The listing builds one solid part. Answer for the finished solid, in the listing's coordinates (mm). A direction names the side the tool comes from. Coordinates: 2 decimals unless noted, no trailing zeros. Loops run counter-clockwise (first coordinate to the right, second up) from the corner with the lowest first, then second, coordinate; pieces in that order, holes last. Notation, with made-up numbers: (85.5, 42.25) -> (137.5, 42.25) arc R15 cw to (137.5, 56.25) -> close; hole circle Ø1 at (48, 68.5). An arc over 180 degrees is marked (long way). Answer in a Markdown table with one row per item.
```python
from build123d import *

# Parameters (mm, degrees)
F0_W     = 38.1
F0_H     = 605.4239357613
F0_H_2   = 901.7
F0_W_2   = 121.1758604333
F0_H_3   = 38.1
F1_DEPTH = 88.9


# Not quite as in the source:
# - a feature names something its author has since deleted; it is built from what else it names


with BuildPart() as f1:
    # F0 (on Front) → F1 (new body)
    with BuildSketch(Plane.XZ):
        Polygon((0, 38.1), (0, 0), (558.8, 0), (558.8, 38.1), (520.7027813, 38.1), (399.5269208667, 38.1), (361.4269208667, 38.1), (218.8134604333, 38.1), (180.7134604333, 38.1), (38.1, 38.1), align=None)
        with Locations((19.05, 340.8119678807)):
            Rectangle(F0_W, F0_H)
        Polygon((520.7027813, 38.1), (558.8, 38.1), (558.8027813, 38.1), (558.8027813, 939.8), (558.8027813, 1181.4738530943), (558.8027813, 1235.3553898208), (558.8027813, 1270), (520.7027813, 1270), (520.7027813, 977.9), (520.7027813, 939.8), align=None)
        Polygon((69.5237996219, 939.8), (0, 643.5239357613), (38.1, 643.5239357613), (39.1349278428, 643.5239357613), (108.6587274647, 939.8), align=None)
        with Locations((199.7634604333, 488.95)):
            Rectangle(F0_W, F0_H_2)
        Polygon((96.2017068277, 977.9), (69.5237996219, 939.8), (108.6587274647, 939.8), (180.7134604333, 939.8), (218.8134604333, 939.8), (361.4269208667, 939.8), (361.4269208667, 977.9), (142.7132186595, 977.9), align=None)
        Polygon((361.4269208667, 38.1), (399.5269208667, 38.1), (399.5269208667, 939.8), (399.5269208667, 977.9), (399.5269208667, 1270), (361.4269208667, 1270), (361.4269208667, 977.9), (361.4269208667, 939.8), align=None)
        with Locations((460.1148510833, 958.85)):
            Rectangle(F0_W_2, F0_H_3)
        Polygon((300.7323287388, 1270), (96.2017068277, 977.9), (142.7132186595, 977.9), (347.2438405706, 1270), align=None)
        Polygon((558.8027813, 1235.3553898208), (558.8027813, 1181.4738530943), (774.3289282057, 1397), (720.4473914792, 1397), align=None)
        Polygon((338.8323287388, 1308.1), (300.7323287388, 1270), (347.2438405706, 1270), (361.4269208667, 1270), (399.5269208667, 1270), (520.7027813, 1270), (558.8027813, 1270), (558.8027813, 1308.1), (520.7027813, 1308.1), (415.0323287388, 1308.1), (339.9874666667, 1308.1), align=None)
        Polygon((720.4473914792, 1397), (774.3289282057, 1397), (965.2027813, 1397), (965.2027813, 1435.1), (558.8027813, 1435.1), (558.8027813, 1397), align=None)
        Polygon((558.8027813, 1435.1), (338.8323287388, 1308.1), (339.9874666667, 1308.1), (415.0323287388, 1308.1), (520.7027813, 1369.1088642316), (558.8027813, 1391.1059094878), (558.8027813, 1397), align=None)
        Polygon((520.7027813, 1308.1), (558.8027813, 1308.1), (558.8027813, 1391.1059094878), (520.7027813, 1369.1088642316), align=None)
    extrude(amount=F1_DEPTH)

    # F2: F1 across face


with BuildPart() as f1_1:
    add(f1.part)
    add(f1.part.mirror(Plane(origin=(965.2027813, -44.45, 1416.05), x_dir=(0, 1, 0), z_dir=(1, 0, 0))))


solid = f1_1.part
```
Item 1: A cutting plane is placed at B-B, the plane z = 1207. Determine the outline of the cut face in (x, y).
Findings below:
| item | result |
|---|---|
| outline | (256.62, -88.9) -> (303.13, -88.9) -> (303.13, 0) -> (256.62, 0) -> close; (361.43, -88.9) -> (399.53, -88.9) -> (399.53, 0) -> (361.43, 0) -> close; (520.7, -88.9) -> (584.33, -88.9) -> (584.33, 0) -> (520.7, 0) -> close; (1346.08, -88.9) -> (1409.7, -88.9) -> (1409.7, 0) -> (1346.08, 0) -> close; (1530.88, -88.9) -> (1568.98, -88.9) -> (1568.98, 0) -> (1530.88, 0) -> close; (1627.27, -88.9) -> (1673.79, -88.9) -> (1673.79, 0) -> (1627.27, 0) -> close |
Item 2: A tool of negligible diameter and unlimited length cuts with its end or side. For faces 5 (the face through (665.06, -43.83, 1287.73)), 6 (the face through (38.1, -44, 337)), 7 (the face through (1895.157, -43.828, 793.736)), from which of +Z, -Z, +X, -X, +Y, -Y can it reach the whole face along a straight path? Write none if from no direction.
Findings below:
| item | result |
|---|---|
| face 5 | -Z, +Y, -Y |
| face 6 | +Y, -Y |
| face 7 | +Z, +X, +Y, -Y |
Item 3: Determine the mould class of faces 1 (the face through (558.803, -44, 602)), 2 (the face through (469, -44, 1308.1)), 3 (the face through (960, -44, 1435.1)), 4 (the face through (1289.65, -43.83, 1317.31)) for opening direction Z: +Z half, -Z half, draft (parallel to the pull), parting line (faces both ways), or undercut.
Findings below:
| item | result |
|---|---|
| face 1 | draft |
| face 2 | undercut |
| face 3 | +Z half |
| face 4 | undercut |
Item 4: Flat-ended cylindrical pins translate along their axes: pin 1 Ø2 at (x, y) = (346.5, -68) entering from +Z; pin 2 Ø2 at (y, z) = (-41, 422) entering from -X; pin 3 Ø1.5 at (y, z) = (-29.5, 854) entering from -X. Find the tip coordinate at first contact, or state that the pin passes through.
Findings below:
| item | result |
|---|---|
| pin 1 | stops at z = 1313.1 |
| pin 2 | stops at x = 0 |
| pin 3 | stops at x = 49.21 |
Item 5: A cutting plane is placed at C-C, the plane x = 1088. Determine the outline of the cut face in (y, z), plus the area to 3 significant figures.
Findings below:
| item | result |
|---|---|
| outline | (-88.9, 1397) -> (0, 1397) -> (0, 1435.1) -> (-88.9, 1435.1) -> close |
| area | 3,390 mm2 |
Item 6: A cutting plane is placed at A-A, the plane z = 337. Count the separate pieces of the cut face and the enclosed holes in it, plus the area to 3 significant figures.
Findings below:
| item | result |
|---|---|
| separate pieces | 8 |
| enclosed holes | 0 |
| area | 27,100 mm2 |
Item 7: Find the intervals of material crossed by probe 1 along X at (y, z) = (-5.5, 1319.5); probe 2 along Z at (x, y) = (257, -63.5); probe 3 along Z at (x, y) = (1454, -79), in increasing order.
Findings below:
| item | result |
|---|---|
| probe 1 | x = 358.58 to 434.78, 520.7 to 558.8, 642.95 to 696.83, 1233.58 to 1287.46, 1371.6 to 1409.7, 1495.63 to 1571.83 |
| probe 2 | z = 0 to 38.1, 939.8 to 977.9, 1141.12 to 1207.54 |
| probe 3 | z = 0 to 38.1, 939.8 to 977.9, 1270 to 1308.1, 1343.53 to 1387.53 |
